```python
from build123d import *

# Parameters (mm, degrees)
SKETCH1_W           = 42.8625
SKETCH1_H           = 42.8625
BOSS_EXTRUDE1_DEPTH = 254
SHELL1_T            = -3.175
BOSS_EXTRUDE2_DEPTH = 21.43125
CIRPATTERN1_START   = -21.43125
CIRPATTERN1_DEPTH   = 42.8625
CIRPATTERN1_2_DEPTH = 42.8625
BOSS_EXTRUDE3_DEPTH = 6.35
SKETCH4_R           = 4.7625
CUT_EXTRUDE1_DEPTH  = 416.95027213
BOSS_EXTRUDE4_DEPTH = 3.175
SKETCH6_R           = 4.7625
CUT_EXTRUDE2_DEPTH  = 402.863889424
FILLET1_R           = 5.08
SHELL3_START        = -18.25625
SHELL3_DEPTH        = 36.5125
SHELL3_2_DEPTH      = 36.5125
SHELL3_START_2      = -24.60625
SHELL3_3_DEPTH      = 6.35


with BuildPart() as part:
    # Sketch1 → Boss-Extrude1 (new body)
    with BuildSketch(Plane(origin=(0, 0, 0), x_dir=(1, 0, 0), z_dir=(0, 1, 0))):
        Rectangle(SKETCH1_W, SKETCH1_H)
    extrude(amount=BOSS_EXTRUDE1_DEPTH)

    # Shell1
    shell1_openings = [part.faces().sort_by_distance(p)[0] for p in [
        (0, 254, 0),
    ]]
    offset(amount=SHELL1_T, openings=shell1_openings, kind=Kind.INTERSECTION)

    # Sketch2 → Boss-Extrude2 (add, symmetric)
    with BuildSketch(Plane.XY):
        Polygon((21.43125, 0), (213.51875, -25.4), (218.609622268, 13.099721526), (21.43125, 39.172894719), align=None)
    extrude(amount=BOSS_EXTRUDE2_DEPTH, both=True)

    # CirPattern1: read off the stored shape, not the designer's step
    # CirPattern1 outline → CirPattern1 (add)
    with BuildSketch(Plane.YZ.offset(CIRPATTERN1_START)):
        Polygon((13.099721526, -218.609622268), (39.172894719, -21.43125), (0, -21.43125), (-25.4, -213.51875), align=None)
        Polygon((-25.4, 213.51875), (0, 21.43125), (39.172894719, 21.43125), (13.099721526, 218.609622268), align=None)
    extrude(amount=CIRPATTERN1_DEPTH)

    # CirPattern1 2 outline → CirPattern1 2 (add)
    with BuildSketch(Plane.XY.offset(CIRPATTERN1_START)):
        Polygon((-213.51875, -25.4), (-21.43125, 0), (-21.43125, 39.172894719), (-218.609622268, 13.099721526), align=None)
    extrude(amount=CIRPATTERN1_2_DEPTH)

    # Sketch3 → Boss-Extrude3 (add)
    with BuildSketch(Plane(origin=(0, 0, -21.43125), x_dir=(-1, 0, 0), z_dir=(0, 0, -1))):
        Polygon((-153.063997925, 1.80984108), (-127.883188972, 5.139534826), (-135.166894041, 60.222554412), (-160.347702995, 56.892860666), align=None)
    extrude(amount=BOSS_EXTRUDE3_DEPTH)

    # Sketch4 → Cut-Extrude1 (cut, through all)
    with BuildSketch(Plane(origin=(0, 0, -27.78125), x_dir=(-1, 0, 0), z_dir=(0, 0, -1))):
        with Locations((-146.092451645, 45.967303062)):
            Circle(SKETCH4_R)
    extrude(amount=-CUT_EXTRUDE1_DEPTH, mode=Mode.SUBTRACT)

    # Sketch5 → Boss-Extrude4 (add, symmetric)
    with BuildSketch(Plane.XY):
        Polygon((161.952802122, 20.591532454), (166.531131023, 55.215144766), (191.711939977, 51.88545102), (187.133611076, 17.261838709), align=None)
    extrude(amount=BOSS_EXTRUDE4_DEPTH, both=True)

    # Sketch6 → Cut-Extrude2 (cut, through all)
    with BuildSketch(Plane.XY.offset(3.175)):
        with Locations((177.456688627, 40.959893416)):
            Circle(SKETCH6_R)
    extrude(amount=-CUT_EXTRUDE2_DEPTH, mode=Mode.SUBTRACT)

    # Fillet1
    fillet1_edges = [part.edges().sort_by_distance(p)[0] for p in [
        (160.347702995, 56.892860666, -24.60625),
        (135.166894041, 60.222554412, -24.60625),
        (191.711939977, 51.88545102, 0),
        (166.531131023, 55.215144766, 0),
    ]]
    fillet(fillet1_edges, radius=FILLET1_R)

    # Shell3: read off the stored shape, not the designer's step
    # Shell3 outline → Shell3 (cut)
    with BuildSketch(Plane.YZ.offset(SHELL3_START)):
        Polygon((9.952120407, -218.19341055), (35.970257339, -21.43125), (3.175, -21.43125), (3.175, -21.640257682), (-22.252398881, -213.934961718), align=None)
        Polygon((3.175, 21.640257682), (3.175, 21.43125), (35.970257339, 21.43125), (9.952120407, 218.19341055), (-22.252398881, 213.934961718), align=None)
    extrude(amount=SHELL3_DEPTH, mode=Mode.SUBTRACT)

    # Shell3 2 outline → Shell3 2 (cut)
    with BuildSketch(Plane.XY.offset(SHELL3_START)):
        Polygon((-21.640257682, 3.175), (-21.43125, 3.175), (-21.43125, 35.970257339), (-218.19341055, 9.952120407), (-213.934961718, -22.252398881), align=None)
        Polygon((21.43125, 35.970257339), (21.43125, 3.175), (21.640257682, 3.175), (213.934961718, -22.252398881), (218.19341055, 9.952120407), align=None)
    extrude(amount=SHELL3_2_DEPTH, mode=Mode.SUBTRACT)

    # Shell3 3 outline → Shell3 3 (cut)
    with BuildSketch(Plane.XY.offset(SHELL3_START_2)):
        Polygon((152.093787046, 18.69256649), (133.208180331, 21.189836799), (131.447001809, 7.870924227), (150.332608524, 5.373653917), align=None)
    extrude(amount=SHELL3_3_DEPTH, mode=Mode.SUBTRACT)


solid = part.part
```
CAD build for the part. Positions are in the model's coordinates, mm. A direction names the side the tool comes from. Coordinates: 2 decimals unless noted, no trailing zeros. Order: outer loops, then holes, each group sorted by start corner. A loop starts at its lowest first (then second) coordinate and runs counter-clockwise, first axis right, second up. Notation, with made-up numbers: (78, 25.5) - (117, 25.5) arc R22 cw to (117, 58.5) - close; hole circle Ø4 at (70.25, 16). An arc over 180 degrees is marked (long way). Use a Markdown table: item, result. Add a question column.
(1) Saw through at B-B (x = -102.5). Give the cut face in (y, z), then the cut area to 3 significant figures.
(2) Saw through at A-A (y = 216). Give the cut face in (x, z).
(3) Flat gauge pins, fed straight in: pin 1 (1.5 mm diameter, centred on x = 126.5, y = 16, fed in from +Z); pin 2 (18.5 mm diameter, centred on y = 169.5, z = 3.5, fed in from -X); pin 3 (14.5 mm diameter, centred on x = 175, y = 29, fed in from +Z) (3 decimals). Where does each tip first touch, or does it go through?
(4) Which spindle directions (+Z, -Z, +X, -X, +Y, -Y) get a long thin tool onto all of the face, cutting with end or side? Do faces 4 (the face through (18.256, 6, 121)), 5 (the face through (0, 0, 0)), 6 (the face through (0, 3.175, 0)), 7 (the face through (-21.431, 6, 121)), 8 (the face through (116.44, -9.36, -0.26)). Say none if no direction does.
(5) Pull direction Y, two halves, no side cores. Call faces 1 (the face through (118, 7, -18.256)), 2 (the face through (-218.362, 11.23, -0.3)), 3 (the face through (177, 36, -3.175)): +Y half, -Y half, draft (parallel to the pull), parting line (faces both ways), or undercut.
(6) Drill centre lines: line 1 along X through (y, z) = (19.5, -38); line 2 along Y through (x, z) = (20, -23.5). Where is each one in solid material? Low to high. Write a range as [from, to].
Solved:
| question | item | result |
|---|---|---|
| 1 | outline | (-10.72, -21.43) - (28.45, -21.43) - (28.45, 21.43) - (-10.72, 21.43) - close; hole (-7.52, -18.26) - (25.25, -18.26) - (25.25, 18.26) - (-7.52, 18.26) - close |
| 1 | area | 483 mm² |
| 2 | outline | (-21.43, -21.43) - (21.43, -21.43) - (21.43, 21.43) - (-21.43, 21.43) - close; hole (-18.26, -18.26) - (18.26, -18.26) - (18.26, 18.26) - (-18.26, 18.26) - close |
| 3 | pin 1 | stops at z = 21.43 |
| 3 | pin 2 | stops at x = -21.43 |
| 3 | pin 3 | stops at z = 3.175 |
| 4 | face 4 | none |
| 4 | face 5 | -Y |
| 4 | face 6 | +Y |
| 4 | face 7 | +Z, -X, +Y, -Y |
| 4 | face 8 | +X |
| 5 | face 1 | undercut |
| 5 | face 2 | -Y half |
| 5 | face 3 | draft |
| 6 | line 1 | x = [-21.43, -18.26], [18.26, 21.43] |
| 6 | line 2 | y = [-0.27, 38.9] |
